Can you work these out from the model? Positions are in its coordinate system, mm. A direction names the side the tool comes from. Round coordinates to 2 decimals unless told otherwise and drop trailing zeros. Write each loop counter-clockwise with the first axis right and the second up, starting at its lowest first coordinate (ties: lowest second). Pieces come first, ordered by that corner, then holes.
Q1. For faces 1 (the flat face through (-4, 6.5, 0)), 2 (the flat face through (-4, 0, -7.5)), which set-ups out of +Z, -Z, +X, -X, +Y, -Y let a thin tool reach every point of the face, with its end or its side?
Q2. If we section it at A-A (y = 3.25): Please give me the cut outline in (x, z).
Q3. We'd pull the mould along Y, two halves only. Please class faces 3 (the flat face through (-4, 7.5, 0)), 4 (the flat face through (-4, -7.5, 0)), 5 (the flat face through (-4, -6.5, 0)): +Y half, -Y half, draft (parallel to the pull), parting line (faces both ways), or undercut.
Q4. I'm going to push a flat-ended pin straight in: pin 1 Ø4.5 at (x, z) = (243.5, 0) entering from +Y. Where does the tip first touch, or does it pass through?
Q5. Please list where these lines run through material, in increasing order: line 1 along Y through (x, z) = (146.5, -4); line 2 along Z through (x, y) = (-243.5, -7.1).
Q6. If we section it at B-B (x = 24): Please give me the cut outline in (y, z).
from build123d import *

# Parameters (mm, degrees)
SKETCH_11_W         = 15
SKETCH_11_H         = 15
SKETCH_11_W_2       = 13
SKETCH_11_H_2       = 13
F_15X15X1_1_DEPTH   = 640
SKETCH_12_R         = 1.95
CUT_EXTRUDE_1_DEPTH = 321.43915179
SKETCH_13_R         = 1.45
CUT_EXTRUDE_2_DEPTH = 321.43915179
SKETCH_14_R         = 1.45
CUT_EXTRUDE_3_DEPTH = 321.43915179
SKETCH_15_W         = 44.103354617
SKETCH_15_H         = 76.02578272
SKETCH_15_W_2       = 30.662332257
SKETCH_15_H_2       = 81.486198053
CUT_EXTRUDE_4_DEPTH = 321.43915179


with BuildPart() as part:
    # 草图11 → 铝管 15X15X1(1) (new body)
    with BuildSketch(Plane(origin=(-320, 0, 0), x_dir=(0, 0, -1), z_dir=(1, 0, 0))):
        Rectangle(SKETCH_11_W, SKETCH_11_H)
        Rectangle(SKETCH_11_W_2, SKETCH_11_H_2, mode=Mode.SUBTRACT)
    extrude(amount=F_15X15X1_1_DEPTH)

    # 草图12 → 切除-拉伸1 (cut, through all)
    with BuildSketch(Plane(origin=(0, 7.5, 0), x_dir=(1, 0, 0), z_dir=(0, 1, 0))):
        with Locations(Location((-41.5, 0, 0), (0, 0, 270))):
            Circle(SKETCH_12_R)
        with Locations(Location((-270, 0, 0), (0, 0, 270))):
            Circle(SKETCH_12_R)
        with Locations(Location((270, 0, 0), (0, 0, 90))):
            Circle(SKETCH_12_R)
        with Locations(Location((41.5, 0, 0), (0, 0, 90))):
            Circle(SKETCH_12_R)
    extrude(amount=-CUT_EXTRUDE_1_DEPTH, mode=Mode.SUBTRACT)

    # 草图13 → 切除-拉伸2 (cut, through all)
    with BuildSketch(Plane(origin=(0, 7.5, 0), x_dir=(1, 0, 0), z_dir=(0, 1, 0))):
        with Locations(Location((-243.5, 0, 0), (0, 0, 270))):
            Circle(SKETCH_13_R)
        with Locations(Location((243.5, 0, 0), (0, 0, 90))):
            Circle(SKETCH_13_R)
    extrude(amount=-CUT_EXTRUDE_2_DEPTH, mode=Mode.SUBTRACT)

    # 草图14 → 切除-拉伸3 (cut, through all)
    with BuildSketch(Plane(origin=(0, 7.5, 0), x_dir=(1, 0, 0), z_dir=(0, 1, 0))):
        with Locations(Location((-16.5, 0, 0), (0, 0, 270))):
            Circle(SKETCH_14_R)
        with Locations(Location((16.5, 0, 0), (0, 0, 270))):
            Circle(SKETCH_14_R)
    extrude(amount=-CUT_EXTRUDE_3_DEPTH, mode=Mode.SUBTRACT)

    # 草图15 → 切除-拉伸4 (cut, through all)
    with BuildSketch(Plane(origin=(0, 7.5, 0), x_dir=(1, 0, 0), z_dir=(0, 1, 0))):
        with Locations((-312.051677309, 7.560575077)):
            Rectangle(SKETCH_15_W, SKETCH_15_H)
        with Locations((305.331166129, -3.150239616)):
            Rectangle(SKETCH_15_W_2, SKETCH_15_H_2)
    extrude(amount=-CUT_EXTRUDE_4_DEPTH, mode=Mode.SUBTRACT)


solid = part.part
A:
1. face 1: +X, -X
1. face 2: -Z, +X, -X, +Y, -Y
2. outline: (-290, -7.5) - (290, -7.5) - (290, -6.5) - (-290, -6.5) - close; (-290, 6.5) - (290, 6.5) - (290, 7.5) - (-290, 7.5) - close
3. face 3: +Y half
3. face 4: -Y half
3. face 5: undercut
4. pin 1: stops at y = 7.5
5. line 1: y = -7.5 to -6.5, 6.5 to 7.5
5. line 2: z = -7.5 to -1.45, 1.45 to 7.5
6. outline: (-7.5, -7.5) - (7.5, -7.5) - (7.5, 7.5) - (-7.5, 7.5) - close; hole (-6.5, -6.5) - (6.5, -6.5) - (6.5, 6.5) - (-6.5, 6.5) - close
